Input: dimensioned drawing with shaded views. Units: mm. Origin: part minimum x, y, z. A direction names the side the tool comes from. Round coordinates to 2 decimals unless told otherwise and drop trailing zeros. Loops run counter-clockwise (first coordinate to the right, second up) from the corner with the lowest first, then second, coordinate; pieces in that order, holes last. Notation, with made-up numbers: M -14.75,-18 L -5.75,-18 A21 cw -5.75,2 Z; hole C 61,-6.75 d2. An arc over 180 degrees is marked long. Write each question's results on one line, items separated by ' | '. Start each with the question number.
1. Set-up query: the marked faces 1 and 2. Return all of +Z, -Z, +X, -X, +Y, -Y with unobstructed straight access to the full face (end or side cutting, diameter ignored); none if empty.
2. Section B-B on y = 4.25. Output: boundary loops of the cut face in (x, z) (1 decimal).
3. Ray query, line 1 (Z direction, x = 5.5, y = 10.75); line 2 (X direction, y = 3.75, z = 17.75); line 3 (X direction, y = 5.5, z = 8.5). Return the intervals inside material, ascending.
4. Section A-A on z = 10. Output: boundary loops of the cut face in (x, y) (1 decimal).
5. Section D-D on z = 14.5. Output: boundary loops of the cut face in (x, y), and give its area (3 significant figures).
6. Section C-C on x = 3.5. Output: boundary loops of the cut face in (y, z).
7. Contact query for flat-ended pins moving along their axis: pin 1 Ø1.2 at (y, z) = (2.5, 6.5) entering from +X; pin 2 Ø7 at (x, z) = (5.42, 10) entering from +Y; pin 3 Ø4.5 at (x, z) = (18.5, 13) entering from -Y. Output: stop coordinate, or through.
8. Draft query along Z for the marked faces 3, 4 and 5. Return one class per face: released by +Z, released by -Z, zero draft, split by the parting line, or undercut.
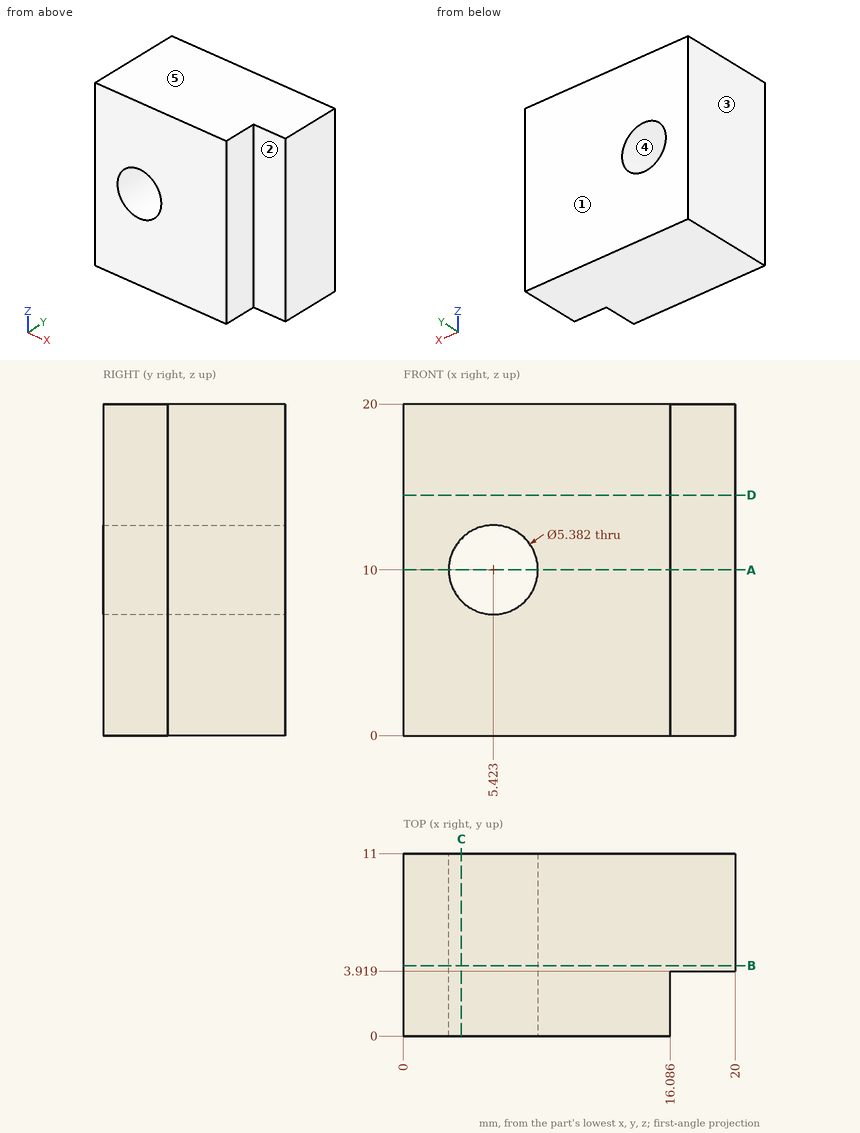
Taken from the geometry:
1) face 1: +Z, -Z, +X, -X, +Y | face 2: +Z, -Z, +X, -Y
2) outline: M 0,0 L 20,0 L 20,20 L 0,20 Z; hole C 5.4,10 d5.4
3) line 1: 0 to 7.31, 12.69 to 20 | line 2: 0 to 16.09 | line 3: 0 to 3.19, 7.66 to 20
4) outline: M 0,0 L 2.7,0 L 2.7,11 L 0,11 Z; M 8.1,0 L 16.1,0 L 16.1,3.9 L 20,3.9 L 20,11 L 8.1,11 Z
5) outline: M 0,0 L 16.09,0 L 16.09,3.92 L 20,3.92 L 20,11 L 0,11 Z | area: 205 mm^2
6) outline: M 0,0 L 11,0 L 11,8.12 L 0,8.12 Z; M 0,11.88 L 11,11.88 L 11,20 L 0,20 Z
7) pin 1: x = 16.09 | pin 2: y = 11 | pin 3: y = 3.92
8) face 3: zero draft | face 4: undercut | face 5: released by +Z
